Read the model definition and answer for the solid it produces. Units are mm, in the model's axes. A direction names the side the tool comes from. Coordinates: 2 decimals unless noted, no trailing zeros. Write each loop counter-clockwise with the first axis right and the second up, starting at its lowest first coordinate (ties: lowest second). Pieces come first, ordered by that corner, then holes.
Item 1: Straight lines are drawn through the part: probe 1 along Y at (x, z) = (27, 0); probe 2 along Y at (x, z) = (13, 7.5); probe 3 along Z at (x, y) = (15.5, -10.5). For each, find the intervals that lie inside material, in ascending order.
Item 2: Section C-C (x = 8) is taken. Give the vertices of the cut face in (y, z).
Item 3: Section A-A (z = 0) is taken. Give the vertices of the cut face in (x, y) (3 decimals), then the cut area to 3 significant figures.
Item 4: Section B-B (y = 0) is taken. Give the vertices of the cut face in (x, z).
Item 5: A tool of negligible diameter and unlimited length cuts with its end or side. For faces 1 (the face through (45.566, 18.135, 0.456)), 2 (the face through (2.54, -1.76, -39.96)), 3 (the face through (40.14, -7.509, 23.846)), 4 (the face through (11.926, 20.472, -4.546)), from which of +Z, -Z, +X, -X, +Y, -Y can it reach the whole face along a straight path? Write none if from no direction.
Item 6: Determine the mould class of faces 5 (the face through (0, -18.3, 9.4)), 6 (the face through (27.185, -12.394, -1.627)), 7 (the face through (15.04, -0.88, -19.98)) for opening direction Y: released by +Y, released by -Y, zero draft, split by the parting line, or undercut.
Item 7: Each of these flat-tipped pins is pushed along its axis until it touches: P1, Ø6, axis at y = 7.5, z = 10.5, coming from the -X side; P2, Ø11, axis at x = 42.1, z = 0, coming from the -Y side; P3, Ø10, axis at x = 21.5, z = 2, coming from the +Y side; P4, Ø15, axis at y = 0, z = 0, coming from the +X side. Where does it stop, or does it pass through?
from build123d import *

# Parameters (mm, degrees)
M8X1_0_TAPPED_HOLE2_D           = 7
M8X1_0_TAPPED_HOLE2_DEPTH       = 19
M8X1_0_TAPPED_HOLE2_CSINK_D     = 8.05
M8X1_0_TAPPED_HOLE2_CSINK_ANGLE = 90
M8X1_0_TAPPED_HOLE2_TIP         = 2.103012167


with BuildPart() as part:
    # Sketch1 → Revolve2 (revolve)
    with BuildSketch(Plane.XY, mode=Mode.PRIVATE) as revolve2_sk:
        Polygon((5, 12.5), (0, 20), (0, 40), (5, 40), (12.279404685, 20), (17.720595315, 20), (25, 40), (30, 40), (30, 25), (50, 25), (50, 12.5), align=None)
    revolve(revolve2_sk.sketch.rotate(Axis((0, 0, 0), (1, 0, 0)), 90), axis=Axis((0, 0, 0), (1, 0, 0)))

    # M8x1.0 Tapped Hole2
    with Locations(Plane(origin=(42.095304981, 25, 0), x_dir=(0, 0, 1), z_dir=(0, 1, 0))):
        with Locations((0, 0)):
            CounterSinkHole(M8X1_0_TAPPED_HOLE2_D / 2, M8X1_0_TAPPED_HOLE2_CSINK_D / 2, depth=M8X1_0_TAPPED_HOLE2_DEPTH, counter_sink_angle=M8X1_0_TAPPED_HOLE2_CSINK_ANGLE)
            with Locations((0, 0, -(M8X1_0_TAPPED_HOLE2_DEPTH + M8X1_0_TAPPED_HOLE2_TIP / 2))):  # 118° drill point
                Cone(0, M8X1_0_TAPPED_HOLE2_D / 2, M8X1_0_TAPPED_HOLE2_TIP, mode=Mode.SUBTRACT)


solid = part.part
Established:
1. probe 1: y = -40 to -12.5, 12.5 to 40
1. probe 2: y = -18.54 to -10, 10 to 18.54
1. probe 3: z = -17.02 to -6.78, 6.78 to 17.02
2. outline: circle Ø63.52 at (0, 0); hole circle Ø25 at (0, 0)
3. outline: (0, -40) - (5, -40) - (12.279, -20) - (17.721, -20) - (25, -40) - (30, -40) - (30, -25) - (50, -25) - (50, -12.5) - (5, -12.5) - (0, -20) - close; (0, 20) - (5, 12.5) - (38.595, 12.5) - (38.595, 24.475) - (38.07, 25) - (30, 25) - (30, 40) - (25, 40) - (17.721, 20) - (12.279, 20) - (5, 40) - (0, 40) - close; (45.595, 12.5) - (50, 12.5) - (50, 25) - (46.12, 25) - (45.595, 24.475) - close
3. area: 1,520 mm2
4. outline: (0, -40) - (5, -40) - (12.28, -20) - (17.72, -20) - (25, -40) - (30, -40) - (30, -25) - (50, -25) - (50, -12.5) - (5, -12.5) - (0, -20) - close; (0, 20) - (5, 12.5) - (50, 12.5) - (50, 25) - (30, 25) - (30, 40) - (25, 40) - (17.72, 20) - (12.28, 20) - (5, 40) - (0, 40) - close
5. face 1: +Y
5. face 2: +X, -X
5. face 3: +X
5. face 4: none
6. face 5: zero draft
6. face 6: undercut
6. face 7: split by the parting line
7. P1: stops at x = 2.73
7. P2: stops at y = -25
7. P3: stops at y = 40
7. P4: passes through
